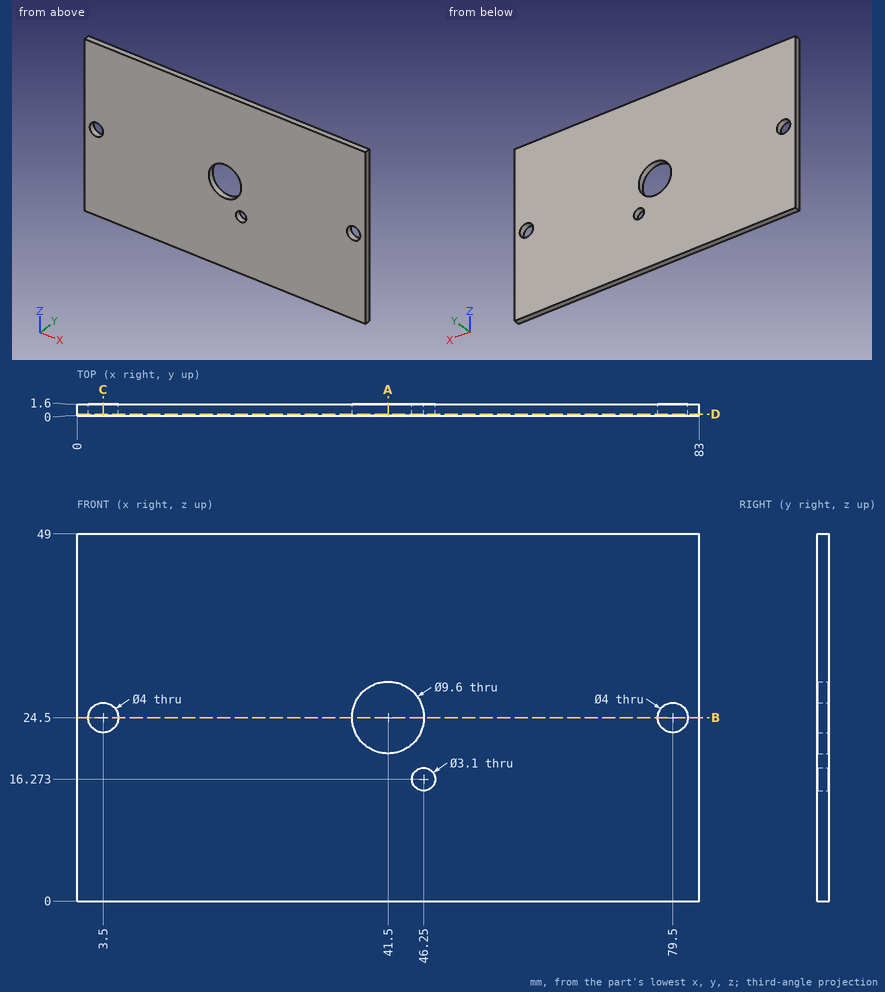
Study the drawing (mm; zero at the part's minimum x, y, z) and answer. Coordinates: 2 decimals unless noted, no trailing zeros. Loops run counter-clockwise (first coordinate to the right, second up) from the corner with the lowest first, then second, coordinate; pieces in that order, holes last. Notation, with made-up numbers: M -10,18.5 L 23,18.5 A15 ccw 23,24.5 Z; hole C 73,63 d11. An arc over 180 degrees is marked long. Answer as a JSON object with one key per item and string values. Group by question number.
Item 1: Each of these flat-tipped pins is pushed along its axis until it touches: P1, Ø5, axis at x = 46.25, z = 16.27, coming from the -Y side; P2, Ø3.5, axis at x = 79.5, z = 24.5, coming from the -Y side. Where does it stop, or does it pass through?
Item 2: Section A-A (x = 41.5) is taken. Write down the section's boundary in (y, z).
Item 3: Section C-C (x = 3.5) is taken. Write down the section's boundary in (y, z), and give its area (3 significant figures).
Item 4: Consider L1, parallel to Z at x = 79.5, y = 0.7; L2, parallel to Z at x = 41.5, y = 1; L3, parallel to X at y = 1.4, z = 16. Determine where each line is inside the solid, lowest interval first.
Item 5: Section D-D (y = 0.25) is taken. Write down the section's boundary in (x, z).
Item 6: Section B-B (z = 24.5) is taken. Write down the section's boundary in (x, y), and give its area (3 significant figures).
Solved:
{
 "1": {"P1": "stops at y = 0", "P2": "passes through"},
 "2": {"outline": "M 0,0 L 1.6,0 L 1.6,19.7 L 0,19.7 Z; M 0,29.3 L 1.6,29.3 L 1.6,49 L 0,49 Z"},
 "3": {"outline": "M 0,0 L 1.6,0 L 1.6,22.5 L 0,22.5 Z; M 0,26.5 L 1.6,26.5 L 1.6,49 L 0,49 Z", "area": "72.0 mm2"},
 "4": {"L1": "z = 0 to 22.5, 26.5 to 49", "L2": "z = 0 to 19.7, 29.3 to 49", "L3": "x = 0 to 44.72, 47.78 to 83"},
 "5": {"outline": "M 0,0 L 83,0 L 83,49 L 0,49 Z; hole C 3.5,24.5 d4; hole C 41.5,24.5 d9.6; hole C 46.25,16.27 d3.1; hole C 79.5,24.5 d4"},
 "6": {"outline": "M 0,0 L 1.5,0 L 1.5,1.6 L 0,1.6 Z; M 5.5,0 L 36.7,0 L 36.7,1.6 L 5.5,1.6 Z; M 46.3,0 L 77.5,0 L 77.5,1.6 L 46.3,1.6 Z; M 81.5,0 L 83,0 L 83,1.6 L 81.5,1.6 Z", "area": "105 mm2"}
}
